Build history of the part. All positions in model axes, mm. Face numbers are marked on the shaded views. A direction names the side the tool comes from. Round coordinates to 2 decimals unless told otherwise and drop trailing zeros. Write each loop counter-clockwise with the first axis right and the second up, starting at its lowest first coordinate (ties: lowest second). Pieces come first, ordered by that corner, then holes. Notation, with made-up numbers: (39, -29) - (52, -29) arc R27 cw to (52, 7) - close; hole circle Ø9 at (-29.5, -0.5). An arc over 180 degrees is marked (long way). Answer as a JSON object with one key per item and string values. Group by question number.
Item 1: Two-plate mould, pull along Y, no slides. Class the marked faces 3, 4 and 5: +Y half, -Y half, draft (parallel to the pull), parting line (faces both ways), or undercut.
Item 2: Probe line 1 (Y direction, x = 21.59, z = 3.1); line 2 (Y direction, x = -42, z = 9); line 3 (Y direction, x = 0, z = 3.3). List the from-to ranges inside material, lowest first. Write a range as from..to.
Item 3: Which spindle directions (+Z, -Z, +X, -X, +Y, -Y) get a long thin tool onto all of the face, cutting with end or side? Do the marked faces 1 and 2. Say none if no direction does.
Item 4: Flat gauge pins, fed straight in: pin 1 (1 mm diameter, centred on y = 14.5, z = 8, fed in from -X); pin 2 (2.5 mm diameter, centred on x = -52.78, y = -28.76, fed in from +Z); pin 3 (6 mm diameter, centred on x = 9.5, y = -23.5, fed in from -Z); pin 4 (1.4 mm diameter, centred on x = 0.5, y = -13, fed in from +Z). Where does each tip first touch, or does it go through?
Item 5: Slice it at C-C, the plane x = 21.59. List the corners of the cut face in (y, z).
Item 6: Slice it at A-A, the plane x = 0. List the corners of the cut face in (y, z), then the cut area to 3 significant figures.
Item 7: Slice it at B-B, the plane y = 12.7. List the corners of the cut face in (x, z), then the cut area to 3 significant figures.
Item 8: Slice it at D-D, the plane y = 2. List the corners of the cut face in (x, z), then the cut area to 3 significant figures.
from build123d import *

# Parameters (mm, degrees)
F1_W      = 111.125
F1_H      = 63.0682
F2_DEPTH  = 1.5875
F3_W      = 111.125
F3_H      = 63.0682
F3_R      = 1.5
F4_DEPTH  = 12.7
F5_R      = 2.38125
F6_W      = 10.5
F6_H      = 5.5245
F6_W_2    = 12.5
F7_DEPTH  = 2.38125
F9_R      = 1.5875
F10_DEPTH = 2.38125
F11_R     = 2.38125
F12_DEPTH = 3.175
F13_R     = 1.190625
F14_DEPTH = 4.7635
F15_R     = 1.5
F16_DEPTH = 14.2885


with BuildPart() as f2:
    # F1 (on Top) → F2 (new body)
    with BuildSketch(Plane.XY):
        Rectangle(F1_W, F1_H)
    extrude(amount=F2_DEPTH)

    # F3 (on face) → F4 (join)
    with BuildSketch(Plane.XY.offset(1.5875)):
        Rectangle(F3_W, F3_H)
        with Locations((-52.784375, -28.755975)):
            Circle(F3_R, mode=Mode.SUBTRACT)
        with Locations((52.784375, -28.755975)):
            Circle(F3_R, mode=Mode.SUBTRACT)
        with BuildLine():
            Line((52.784375, 25.97785), (53.18125, 25.97785))
            Line((53.18125, 25.97785), (53.18125, -25.97785))
            Line((53.18125, -25.97785), (52.784375, -25.97785))
            ThreePointArc((52.784375, -25.97785), (50.819944, -26.791544), (50.00625, -28.755975))
            Line((50.00625, -28.755975), (50.00625, -29.15285))
            Line((50.00625, -29.15285), (-50.00625, -29.15285))
            Line((-50.00625, -29.15285), (-50.00625, -28.755975))
            ThreePointArc((-50.00625, -28.755975), (-50.819944, -26.791544), (-52.784375, -25.97785))
            Line((-52.784375, -25.97785), (-53.18125, -25.97785))
            Line((-53.18125, -25.97785), (-53.18125, 25.97785))
            Line((-53.18125, 25.97785), (-52.784375, 25.97785))
            ThreePointArc((-52.784375, 25.97785), (-50.819944, 26.791544), (-50.00625, 28.755975))
            Line((-50.00625, 28.755975), (-50.00625, 29.15285))
            Line((-50.00625, 29.15285), (50.00625, 29.15285))
            Line((50.00625, 29.15285), (50.00625, 28.755975))
            ThreePointArc((50.00625, 28.755975), (50.819944, 26.791544), (52.784375, 25.97785))
        make_face(mode=Mode.SUBTRACT)
        with Locations((-52.784375, 28.755975)):
            Circle(F3_R, mode=Mode.SUBTRACT)
        with Locations((52.784375, 28.755975)):
            Circle(F3_R, mode=Mode.SUBTRACT)
    extrude(amount=F4_DEPTH)

    # F5
    f5_edges = [f2.edges().sort_by_distance(p)[0] for p in [
        (55.5625, -31.5341, 7.14375),
        (55.5625, 31.5341, 7.14375),
        (-55.5625, -31.5341, 7.14375),
        (-55.5625, 31.5341, 7.14375),
    ]]
    fillet(f5_edges, radius=F5_R)

    # F6 (on face) → F7 (cut, through all)
    with BuildSketch(Plane.YZ.offset(55.5625)):
        with Locations((-18.5216, 11.52525)):
            Rectangle(F6_W, F6_H)
        with Locations((11.7716, 11.52525)):
            Rectangle(F6_W_2, F6_H)
    extrude(amount=-F7_DEPTH, mode=Mode.SUBTRACT)

    # F9 (on face) → F10 (cut, through all)
    with BuildSketch(Plane(origin=(-55.5625, 0, 0), x_dir=(0, -1, 0), z_dir=(-1, 0, 0))):
        Polygon((19.05, 14.2875), (-19.05, 14.2875), (-20.955, 3.4925), (20.955, 3.4925), align=None)
        with Locations((-23.495, 8.89)):
            Circle(F9_R)
        with Locations((23.495, 8.89)):
            Circle(F9_R)
    extrude(amount=-F10_DEPTH, mode=Mode.SUBTRACT)

    # F11 (on face) → F12 (join)
    with BuildSketch(Plane.XY.offset(1.5875)):
        with Locations((0, 12.7)):
            Circle(F11_R)
        with Locations((0, -12.7)):
            Circle(F11_R)
        with Locations((21.59, -12.7)):
            Circle(F11_R)
    extrude(amount=F12_DEPTH)

    # F13 (on face) → F14 (cut, through all)
    with BuildSketch(Plane.XY.offset(4.7625)):
        with Locations((0, 12.7)):
            Circle(F13_R)
        with Locations((0, -12.7)):
            Circle(F13_R)
        with Locations((21.59, -12.7)):
            Circle(F13_R)
    extrude(amount=-F14_DEPTH, mode=Mode.SUBTRACT)

    # F15 (on face) → F16 (cut, through all)
    with BuildSketch(Plane.XY.offset(14.2875)):
        with Locations((52.784375, 28.755975)):
            Circle(F15_R)
        with Locations((52.784375, -28.755975)):
            Circle(F15_R)
        with Locations((-52.784375, -28.755975)):
            Circle(F15_R)
        with Locations((-52.784375, 28.755975)):
            Circle(F15_R)
    extrude(amount=-F16_DEPTH, mode=Mode.SUBTRACT)


solid = f2.part
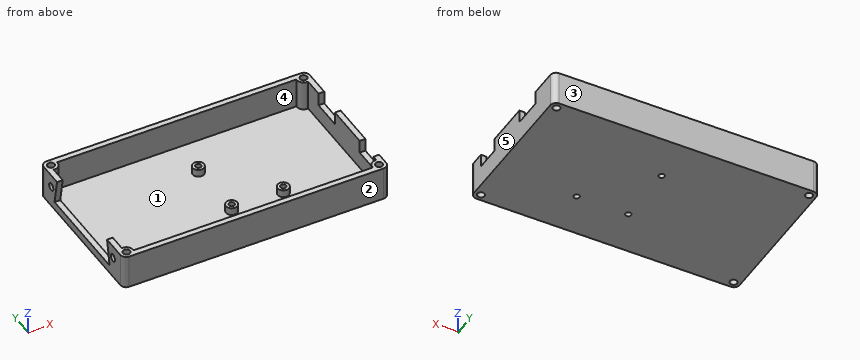
Geometry says:
{
 "1": {"face 3": "+Y half", "face 4": "undercut", "face 5": "draft"},
 "2": {"line 1": "y = -31.53..-29.15, -15.08..-13.89, -11.51..-10.32, 29.15..31.53", "line 2": "y = -31.53..-29.15, 29.15..31.53", "line 3": "y = -31.53..-29.15, -15.08..-13.89, -11.51..-10.32, 10.32..11.51, 13.89..15.08, 29.15..31.53"},
 "3": {"face 1": "+Z", "face 2": "+Z, -Z, +X, -X, -Y"},
 "4": {"pin 1": "stops at x = 53.18", "pin 2": "passes through", "pin 3": "stops at z = 0", "pin 4": "stops at z = 4.76"},
 "5": {"outline": "(-31.53, 0) - (-13.89, 0) - (-13.89, 4.76) - (-15.08, 4.76) - (-15.08, 1.59) - (-29.15, 1.59) - (-29.15, 14.29) - (-31.53, 14.29) - close; (-11.51, 0) - (31.53, 0) - (31.53, 14.29) - (29.15, 14.29) - (29.15, 1.59) - (-10.32, 1.59) - (-10.32, 4.76) - (-11.51, 4.76) - close"},
 "6": {"outline": "(-31.53, 0) - (-13.89, 0) - (-13.89, 4.76) - (-15.08, 4.76) - (-15.08, 1.59) - (-29.15, 1.59) - (-29.15, 14.29) - (-31.53, 14.29) - close; (-11.51, 0) - (11.51, 0) - (11.51, 4.76) - (10.32, 4.76) - (10.32, 1.59) - (-10.32, 1.59) - (-10.32, 4.76) - (-11.51, 4.76) - close; (13.89, 0) - (31.53, 0) - (31.53, 14.29) - (29.15, 14.29) - (29.15, 1.59) - (15.08, 1.59) - (15.08, 4.76) - (13.89, 4.76) - close", "area": "168 mm^2"},
 "7": {"outline": "(-55.56, 0) - (-1.19, 0) - (-1.19, 4.76) - (-2.38, 4.76) - (-2.38, 1.59) - (-53.18, 1.59) - (-53.18, 3.49) - (-55.56, 3.49) - close; (1.19, 0) - (55.56, 0) - (55.56, 8.76) - (53.18, 8.76) - (53.18, 1.59) - (2.38, 1.59) - (2.38, 4.76) - (1.19, 4.76) - close", "area": "202 mm^2"},
 "8": {"outline": "(-55.56, 0) - (55.56, 0) - (55.56, 14.29) - (53.18, 14.29) - (53.18, 1.59) - (-53.18, 1.59) - (-53.18, 3.49) - (-55.56, 3.49) - close", "area": "211 mm^2"}
}
